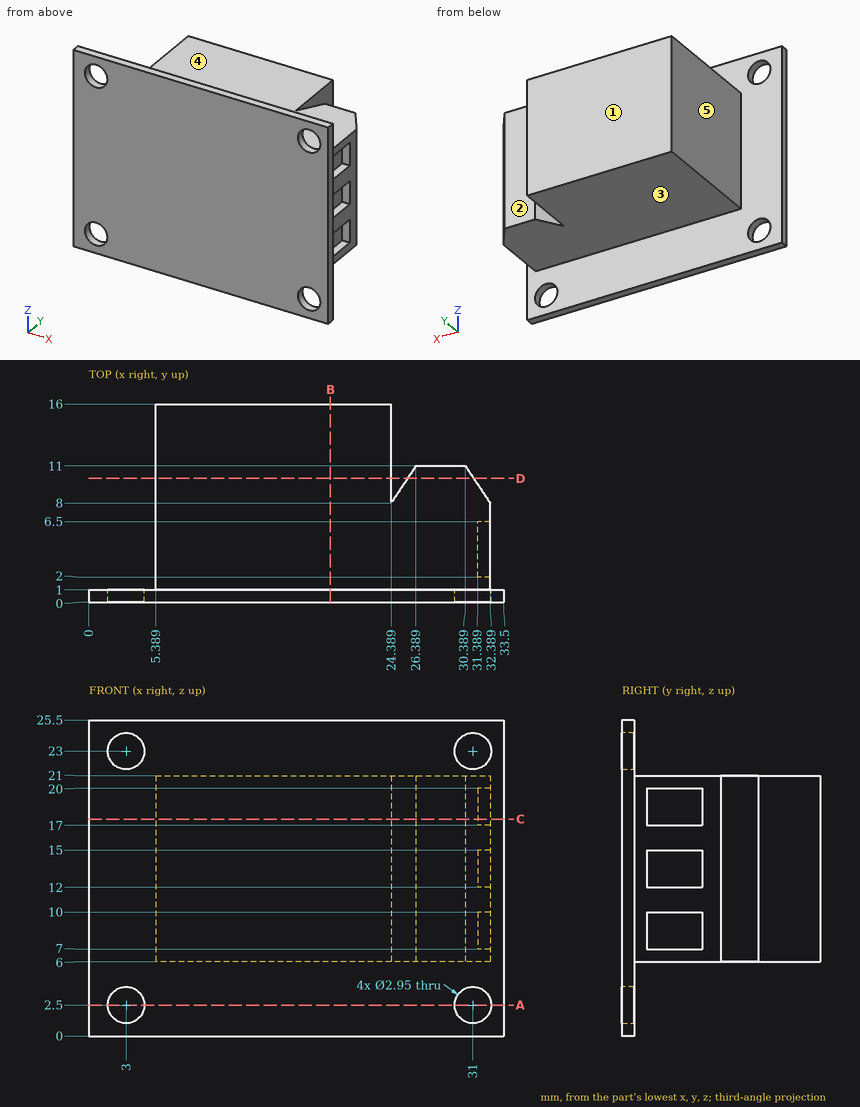
Answer from the drawing. Dimensions are ordinates in mm from the lowest x, y and z of the part. A direction names the side the tool comes from. Coordinates: 2 decimals unless noted, no trailing zeros. Write each loop counter-clockwise with the first axis right and the second up, starting at its lowest first coordinate (ties: lowest second). Pieces come first, ordered by that corner, then holes. Notation, with made-up numbers: (24.25, 87.25) - (46.25, 87.25) arc R27 ccw to (46.25, 113.25) - close; hole circle Ø7 at (12, -7). An arc over 180 degrees is marked (long way). Return JSON: item names as keys, results as strings. Group by question number.
Q1. The part is cut by section A-A on z = 2.5. Write down the section's boundary in (x, y) (1 decimal).
Q2. Which of the six approach directions +Z, -Z, +X, -X, +Y, -Y give full straight-line access (tool end or side, diameter ignored) to the marked faces 1, 2, 3, 4 and 5?
Q3. The part is cut by section C-C on z = 17.5. Write down the section's boundary in (x, y), and give its area (3 significant figures).
Q4. The part is cut by section B-B on x = 19.5. Write down the section's boundary in (y, z).
Q5. Find the intervals of material crossed by line 1 along X through (y, z) = (0.65, 2.5) (1 decimal); line 2 along Z through (x, y) = (32, 5.25); line 3 along Y through (x, z) = (20.5, 23.5), in increasing order. Write a range as [from, to].
Q6. The part is cut by section D-D on y = 10. Write down the section's boundary in (x, z).
Q7. Flat-ended cylindrical pins translate along their axes: pin 1 Ø3.5 at (x, z) = (31, 2.5) entering from -Y; pin 2 Ø1.5 at (y, z) = (5.5, 18) entering from +X; pin 3 Ø2 at (y, z) = (9, 20.5) entering from -X; pin 4 Ø6 at (x, y) = (19.5, 4.5) entering from +Z. Find the tip coordinate at first contact, or state that the pin passes through.
Evaluation:
{
 "1": {"outline": "(0, 0) - (1.5, 0) - (1.5, 1) - (0, 1) - close; (4.5, 0) - (29.5, 0) - (29.5, 1) - (4.5, 1) - close; (32.5, 0) - (33.5, 0) - (33.5, 1) - (32.5, 1) - close"},
 "2": {"face 1": "+Z, -Z, +X, -X, +Y", "face 2": "+Z, -Z, +X, +Y", "face 3": "-Z, +X, -X, +Y", "face 4": "+Z, +X, -X, +Y", "face 5": "+Z, -Z, -X, +Y"},
 "3": {"outline": "(0, 0) - (33.5, 0) - (33.5, 1) - (32.39, 1) - (32.39, 2) - (31.39, 2) - (31.39, 6.5) - (32.39, 6.5) - (32.39, 8) - (30.39, 11) - (26.39, 11) - (24.39, 8) - (24.39, 16) - (5.39, 16) - (5.39, 1) - (0, 1) - close", "area": "388 mm2"},
 "4": {"outline": "(0, 0) - (1, 0) - (1, 6) - (16, 6) - (16, 21) - (1, 21) - (1, 25.5) - (0, 25.5) - close"},
 "5": {"line 1": "x = [0, 1.5], [4.5, 29.5], [32.5, 33.5]", "line 2": "z = [6, 7], [10, 12], [15, 17], [20, 21]", "line 3": "y = [0, 1]"},
 "6": {"outline": "(5.39, 6) - (24.39, 6) - (24.39, 21) - (5.39, 21) - close; (25.72, 6) - (31.06, 6) - (31.06, 21) - (25.72, 21) - close"},
 "7": {"pin 1": "stops at y = 0", "pin 2": "stops at x = 31.39", "pin 3": "stops at x = 5.39", "pin 4": "stops at z = 21"}
}
